Check sheet for the drawn part. Datum: minimum x, y, z corner. Units: mm. A direction names the side the tool comes from. Give positions to 0.01 mm unless a question says otherwise; leave off trailing zeros. Write each loop counter-clockwise with the first axis right and the second up, starting at its lowest first coordinate (ties: lowest second). Pieces come first, ordered by that corner, then holes.
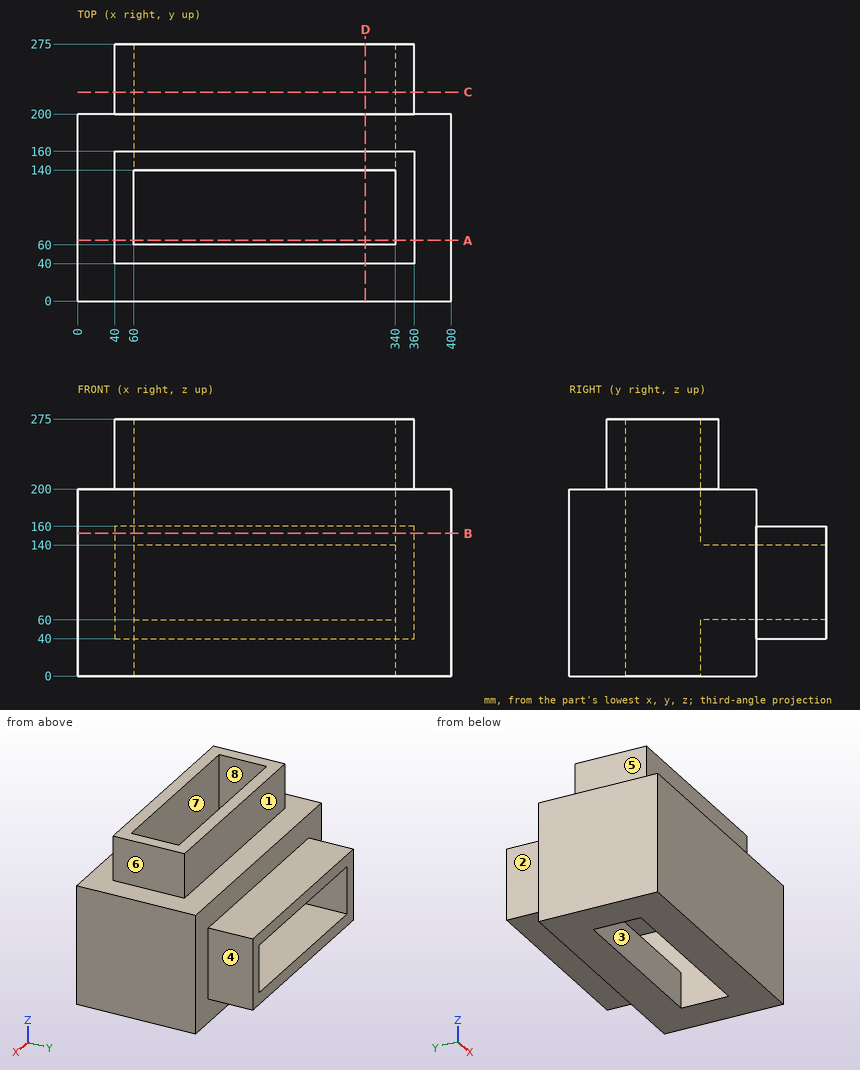
1) Sectioned sample at D-D on x = 308. Record the boundary of the cut face in (y, z), then the cut area to 3 significant figures.
2) Scan lines: L1, parallel to Z at x = 104.5, y = 258.5; L2, parallel to Y at x = 152.5, z = 143.5; L3, parallel to X at y = 71.5, z = 203. Record each from-to range of solid material in increasing order.
3) Sectioned sample at A-A on y = 65. Record the boundary of the cut face in (x, z).
4) Sectioned sample at B-B on z = 152.5. Record the boundary of the cut face in (x, y), then the cut area to 3 significant figures.
5) Draft check along Y on the marked faces 1, 2 and 3. Enter one of: +Y half, -Y half, draft (parallel to the pull), parting line (faces both ways), or undercut.
6) Sectioned sample at C-C on y = 223.5. Record the boundary of the cut face in (x, z).
7) Access from +Z, -Z, +X, -X, +Y, -Y to the whole of each face (thin tool, end or side, straight path). Record for the marked faces 4, 5, 6, 7 and 8.
8) Gauge pin test, flat ends, axial feed: pin 1 (1.5 mm diameter, centred on y = 53, z = 219, fed in from -X); pin 2 (6 mm diameter, centred on y = 222, z = 158.5, fed in from +X); pin 3 (1 mm diameter, centred on x = 268.5, z = 237, fed in from -Y). Record the tip position at first contact, or that the pin passes through.
Answers below:
1. outline: (0, 0) - (60, 0) - (60, 275) - (40, 275) - (40, 200) - (0, 200) - close; (140, 0) - (200, 0) - (200, 40) - (275, 40) - (275, 60) - (140, 60) - close; (140, 140) - (275, 140) - (275, 160) - (200, 160) - (200, 200) - (160, 200) - (160, 275) - (140, 275) - close
1. area: 25,200 mm2
2. L1: z = 40 to 60, 140 to 160
2. L2: y = 0 to 60, 140 to 275
2. L3: x = 40 to 60, 340 to 360
3. outline: (0, 0) - (60, 0) - (60, 275) - (40, 275) - (40, 200) - (0, 200) - close; (340, 0) - (400, 0) - (400, 200) - (360, 200) - (360, 275) - (340, 275) - close
4. outline: (0, 0) - (400, 0) - (400, 200) - (360, 200) - (360, 275) - (40, 275) - (40, 200) - (0, 200) - close; hole (60, 60) - (340, 60) - (340, 140) - (60, 140) - close
4. area: 81,600 mm2
5. face 1: +Y half
5. face 2: draft
5. face 3: undercut
6. outline: (40, 40) - (360, 40) - (360, 160) - (40, 160) - close; hole (60, 60) - (340, 60) - (340, 140) - (60, 140) - close
7. face 4: +Z, -Z, +X, +Y
7. face 5: +Z, -X, +Y, -Y
7. face 6: +Z, +X, +Y, -Y
7. face 7: +Z, -Z
7. face 8: none
8. pin 1: stops at x = 40
8. pin 2: stops at x = 360
8. pin 3: stops at y = 40
